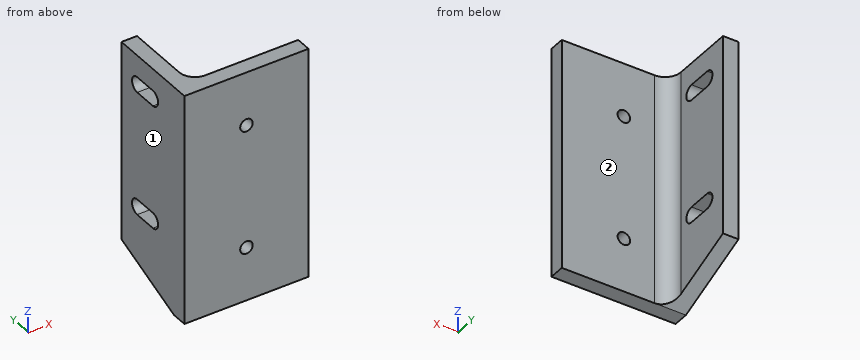
from build123d import *

# Parameters (mm, degrees)
BOSS_EXTRUDE1_DEPTH    = 74.6
CUT_EXTRUDE2_DEPTH     = 87.251900849
CUT_EXTRUDE3_DEPTH     = 10
FILLET1_R              = 5.08
F_10_32_TAPPED_HOLE1_D = 4.0386


with BuildPart() as part:
    # Sketch1 → Boss-Extrude1 (new body)
    with BuildSketch(Plane.XY):
        Polygon((0, 25.48), (0, 0), (35, 0), (35, -5), (-5, -5), (-5, 25.48), align=None)
    extrude(amount=BOSS_EXTRUDE1_DEPTH)

    # Sketch3 → Cut-Extrude2 (cut, through all)
    with BuildSketch(Plane(origin=(0, 0, 0), x_dir=(0, 0, -1), z_dir=(1, 0, 0))):
        with BuildLine():
            Line((-67.5, 10.24), (-67.5, 17.86))
            ThreePointArc((-67.5, 17.86), (-65, 20.36), (-62.5, 17.86))
            Line((-62.5, 17.86), (-62.5, 10.24))
            ThreePointArc((-62.5, 10.24), (-65, 7.74), (-67.5, 10.24))
        make_face()
        with BuildLine():
            Line((-27.5, 10.24), (-27.5, 17.86))
            ThreePointArc((-27.5, 17.86), (-25, 20.36), (-22.5, 17.86))
            Line((-22.5, 17.86), (-22.5, 10.24))
            ThreePointArc((-22.5, 10.24), (-25, 7.74), (-27.5, 10.24))
        make_face()
    extrude(amount=-CUT_EXTRUDE2_DEPTH, mode=Mode.SUBTRACT)

    # Sketch4 → Cut-Extrude3 (cut)
    with BuildSketch(Plane(origin=(0, 0, 0), x_dir=(0, 0, -1), z_dir=(1, 0, 0))):
        Polygon((-10, 25.48), (0, 0), (0, 25.48), align=None)
    extrude(amount=-CUT_EXTRUDE3_DEPTH, mode=Mode.SUBTRACT)

    # Fillet1
    fillet1_edges = [part.edges().sort_by_distance(p)[0] for p in [
        (0, 0, 37.3),
    ]]
    fillet(fillet1_edges, radius=FILLET1_R)

    # #10-32 Tapped Hole1 (through all)
    with Locations(Plane(origin=(0, 0, 0), x_dir=(1, 0, 0), z_dir=(0, 1, 0))):
        with Locations((15, -17.3), (15, -57.3)):
            Hole(F_10_32_TAPPED_HOLE1_D / 2)


solid = part.part
Here's how the part is built. I have some questions about the finished solid (model axes, mm). Face numbers are marked on the shaded views. A direction names the side the tool comes from. Coordinates: 2 decimals unless noted, no trailing zeros. Write each loop counter-clockwise with the first axis right and the second up, starting at its lowest first coordinate (ties: lowest second). Pieces come first, ordered by that corner, then holes.
1) If we section it at A-A (x = -1.5): List the corners of the cut face in (y, z) for me, plus the area to 3 significant figures.
Filled in:
outline: (-5, 0) - (0, 0) - (25.48, 10) - (25.48, 74.6) - (-5, 74.6) - close; hole (10.24, 22.5) - (17.86, 22.5) arc R2.5 ccw to (17.86, 27.5) - (10.24, 27.5) arc R2.5 ccw to start; hole (10.24, 62.5) - (17.86, 62.5) arc R2.5 ccw to (17.86, 67.5) - (10.24, 67.5) arc R2.5 ccw to start
area: 2,030 mm2
2) I'm going to push flat-ended pins straight in: pin 1 (1.5 mm diameter, centred on y = 12.5, z = 47, fed in from +X); pin 2 (3.5 mm diameter, centred on x = 15, z = 17.3, fed in from +Y); pin 3 (12 mm diameter, centred on x = 30, z = 9.5, fed in from +Y); pin 4 (6 mm diameter, centred on y = 7, z = 11.5, fed in from +X). Where does each tip first touch, or does it pass through?
Filled in:
pin 1: stops at x = 0
pin 2: passes through
pin 3: stops at y = 0
pin 4: stops at x = 0.12
3) If we section it at B-B (z = 65): List the corners of the cut face in (x, y) for me, plus the area to 3 significant figures.
Filled in:
outline: (-5, -5) - (35, -5) - (35, 0) - (5.08, 0) arc R5.08 cw to (0, 5.08) - (0, 7.74) - (-5, 7.74) - close; (-5, 20.36) - (0, 20.36) - (0, 25.48) - (-5, 25.48) - close
area: 270 mm2
4) Which directions (+Z, -Z, +X, -X, +Y, -Y) give clear straight access to the entire face, cutting with the end or side of a thin tool? Please do the marked faces 1 and 2.
Filled in:
face 1: +Z, -Z, -X, +Y, -Y
face 2: +Z, -Z, +X, +Y
5) If I drill on line 1 (Z direction, x = 15, y = -1); line 2 (X direction, y = -1.3, z = 17.3); line 3 (X direction, y = 8, z = 57), over which ranges is the centre line in solid material (lowest first)?
Filled in:
line 1: z = 0 to 15.28, 19.32 to 55.28, 59.32 to 74.6
line 2: x = -5 to 12.98, 17.02 to 35
line 3: x = -5 to 0
6) If we section it at C-C (x = 15): List the corners of the cut face in (y, z) for me, plus the area to 3 significant figures.
Filled in:
outline: (-5, 0) - (0, 0) - (0, 15.28) - (-5, 15.28) - close; (-5, 19.32) - (0, 19.32) - (0, 55.28) - (-5, 55.28) - close; (-5, 59.32) - (0, 59.32) - (0, 74.6) - (-5, 74.6) - close
area: 333 mm2
7) If we section it at D-D (z = 17.3): List the corners of the cut face in (x, y) for me, plus the area to 3 significant figures.
Filled in:
outline: (-5, -5) - (12.98, -5) - (12.98, 0) - (5.08, 0) arc R5.08 cw to (0, 5.08) - (0, 25.48) - (-5, 25.48) - close; (17.02, -5) - (35, -5) - (35, 0) - (17.02, 0) - close
area: 313 mm2
